Print and shaded views of the part. All mm, measured from the part's lowest x, y and z. A direction names the side the tool comes from. Coordinates: 2 decimals unless noted, no trailing zeros. Order: outer loops, then holes, each group sorted by start corner. A loop starts at its lowest first (then second) coordinate and runs counter-clockwise, first axis right, second up. Notation, with made-up numbers: M 63,6.5 L 95,6.5 A21 ccw 95,38.5 Z; hole C -33,-3 d3. An arc over 180 degrees is marked long. Use a Markdown table: item, result. Add a question column.
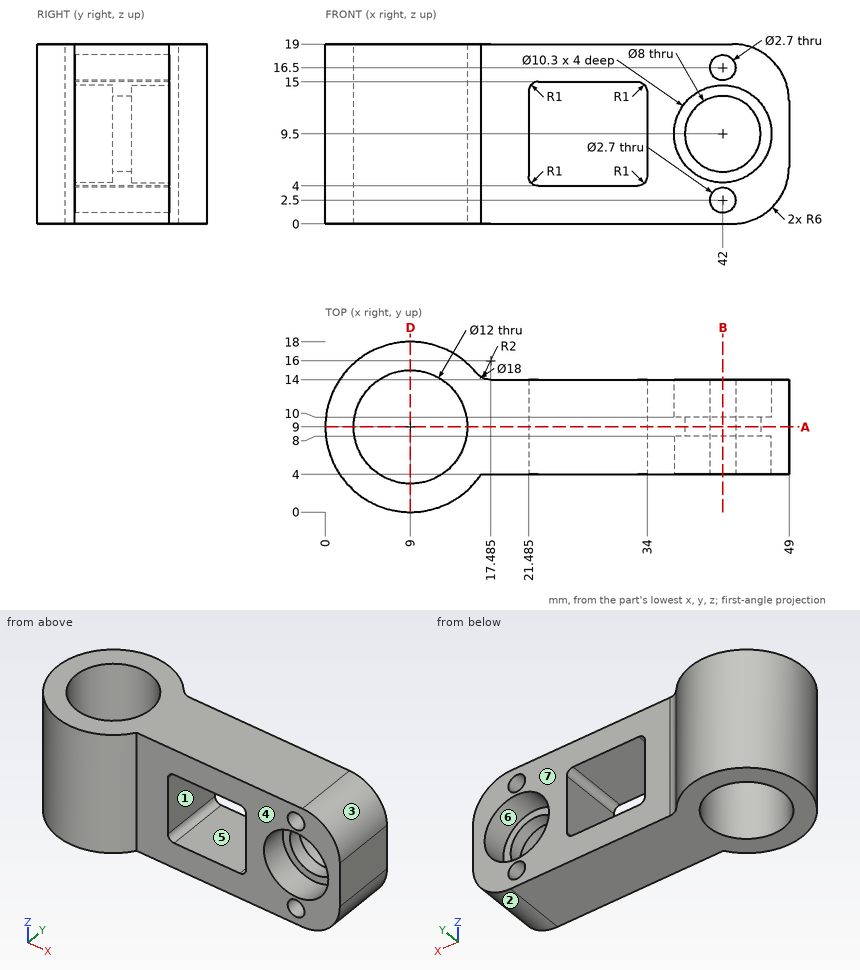
(1) Which spindle directions (+Z, -Z, +X, -X, +Y, -Y) get a long thin tool onto all of the face, cutting with end or side? Do the marked faces 4, 5, 6 and 7. Say none if no direction does.
(2) Mould opens along Z. For the marked faces 1, 2 and 3 say: released by +Z, released by -Z, zero draft, split by the parting line, or undercut.
(3) Drill centre lines: line 1 along Z through (x, y) = (42, 12.45); line 2 along Z through (x, y) = (42, 8.7); line 3 along X through (y, z) = (11.25, 7.25) (1 decimal). Where is each one in solid material? Low to high. Write a range as from..to.
(4) Slice it at B-B on x = 42. Give the cut face in (y, z).
(5) Drop flat-ended pins along their axis: P1, Ø8, axis at x = 40.5, z = 10, coming from the -Y side; P2, Ø4, axis at x = 12, z = 16.5, coming from the +Y side; P3, Ø9.5, axis at x = 42, z = 9.5, coming from the -Y side. Give the stop position or say it passes through.
(6) Slice it at A-A on y = 9. State how many separate pieces and enclosed holes the cut face has, and give its area (3 significant figures).
(7) Slice it at D-D on x = 9. Give the cut face in (y, z), and give its area (3 significant figures).
Solutions:
| question | item | result |
|---|---|---|
| 1 | face 4 | +Z, -Z, +X, -Y |
| 1 | face 5 | +Y, -Y |
| 1 | face 6 | +Y |
| 1 | face 7 | +Z, -Z, +X, +Y |
| 2 | face 1 | undercut |
| 2 | face 2 | released by -Z |
| 2 | face 3 | released by +Z |
| 3 | line 1 | 0..1.15, 3.85..4.35, 14.65..15.15, 17.85..19 |
| 3 | line 2 | 0..1.15, 3.85..5.5, 13.5..15.15, 17.85..19 |
| 3 | line 3 | 0.3..3.4, 14.6..21.5, 34..37.4, 46.6..49 |
| 4 | outline | M 4,0 L 14,0 L 14,1.15 L 4,1.15 Z; M 4,3.85 L 14,3.85 L 14,4.35 L 10,4.35 L 10,5.5 L 8,5.5 L 8,4.35 L 4,4.35 Z; M 4,14.65 L 8,14.65 L 8,13.5 L 10,13.5 L 10,14.65 L 14,14.65 L 14,15.15 L 4,15.15 Z; M 4,17.85 L 14,17.85 L 14,19 L 4,19 Z |
| 5 | P1 | y = 4 |
| 5 | P2 | y = 17.94 |
| 5 | P3 | y = 8 |
| 6 | separate pieces | 2 |
| 6 | enclosed holes | 4 |
| 6 | area | 489 mm² |
| 7 | outline | M 0,0 L 3,0 L 3,19 L 0,19 Z; M 15,0 L 18,0 L 18,19 L 15,19 Z |
| 7 | area | 114 mm² |
